from build123d import *

# Parameters (mm, degrees)
SKETCH3_R           = 145
SKETCH3_R_2         = 105
BOSS_EXTRUDE1_START = -50
SKETCH4_W           = 360
SKETCH4_H           = 360
SKETCH4_R           = 145
BOSS_EXTRUDE1_DEPTH = 50
FILLET1_R           = 20
SKETCH6_W           = 360
SKETCH6_H           = 360
SKETCH6_R           = 145
BOSS_EXTRUDE2_DEPTH = 50
FILLET2_R           = 20
SKETCH7_R           = 30
BOSS_EXTRUDE4_DEPTH = 10


with BuildPart() as part:
    # Sweep-Thin1: sweep along a path in Sketch2
    with BuildLine(Plane.XY) as sweep_thin1_path:
        Line((0, 0), (-150, 0))
        ThreePointArc((-150, 0), (-333.847763109, 76.152236891), (-410, 260))
        Line((-410, 260), (-410, 410))
    # Sketch3 → Sweep-Thin1 (sweep)
    with BuildSketch(Plane(origin=(0, 0, 0), x_dir=(0, 0, -1), z_dir=(1, 0, 0))):
        Circle(SKETCH3_R)
        Circle(SKETCH3_R_2, mode=Mode.SUBTRACT)
    sweep(path=sweep_thin1_path.line)

    # Sketch4 → Boss-Extrude1 (add)
    with BuildSketch(Plane(origin=(0, 0, 0), x_dir=(0, 0, -1), z_dir=(1, 0, 0)).offset(BOSS_EXTRUDE1_START)):
        Rectangle(SKETCH4_W, SKETCH4_H)
        with Locations(Location((0, 0, 0), (0, 0, 270))):
            Circle(SKETCH4_R, mode=Mode.SUBTRACT)
    extrude(amount=BOSS_EXTRUDE1_DEPTH)

    # Fillet1
    fillet1_edges = [part.edges().sort_by_distance(p)[0] for p in [
        (-25, -180, -180),
        (-25, -180, 180),
        (-25, 180, 180),
        (-25, 180, -180),
    ]]
    fillet(fillet1_edges, radius=FILLET1_R)

    # Sketch6 → Boss-Extrude2 (add)
    with BuildSketch(Plane(origin=(0, 410, 0), x_dir=(1, 0, 0), z_dir=(0, 1, 0))):
        with Locations((-410, 0)):
            Rectangle(SKETCH6_W, SKETCH6_H)
        with Locations(Location((-410, 0, 0), (0, 0, 180))):
            Circle(SKETCH6_R, mode=Mode.SUBTRACT)
    extrude(amount=-BOSS_EXTRUDE2_DEPTH)

    # Fillet2
    fillet2_edges = [part.edges().sort_by_distance(p)[0] for p in [
        (-230, 385, 180),
        (-590, 385, 180),
        (-590, 385, -180),
        (-230, 385, -180),
    ]]
    fillet(fillet2_edges, radius=FILLET2_R)

    # Sketch7 → Boss-Extrude4 (add)
    with BuildSketch(Plane(origin=(0, 0, 0), x_dir=(0, 0, -1), z_dir=(1, 0, 0))):
        with Locations((-130, 130)):
            Circle(SKETCH7_R)
    extrude(amount=-BOSS_EXTRUDE4_DEPTH)


solid = part.part
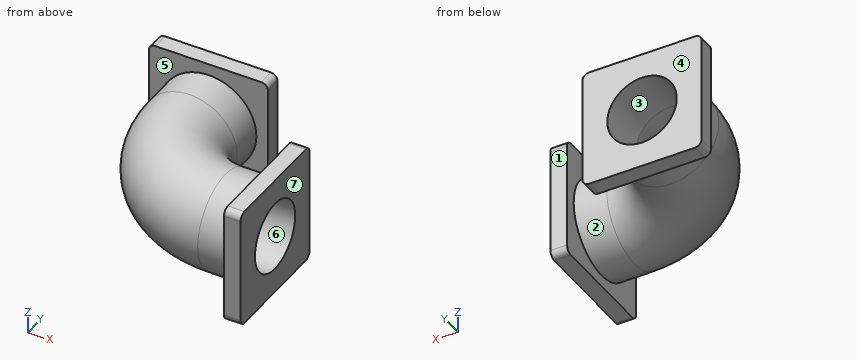
Can you work these out from the model? Positions are in its coordinate system, mm. Face numbers are marked on the shaded views. A direction names the side the tool comes from. Round coordinates to 2 decimals unless told otherwise and drop trailing zeros. Order: outer loops, then holes, each group sorted by start corner. A loop starts at its lowest first (then second) coordinate and runs counter-clockwise, first axis right, second up. Notation, with made-up numbers: (87.5, -33) -> (96.5, -33) arc R14 cw to (96.5, -17) -> close; hole circle Ø3 at (46.5, -38). An arc over 180 degrees is marked (long way). Write each question's results on one line, items separated by ' | '. Start each with the question number.
Item 1: Which directions (+Z, -Z, +X, -X, +Y, -Y) give clear straight access to the entire face, cutting with the end or side of a thin tool? Please do the marked faces 1, 2 and 3.
Item 2: Will these pins go through, and if not, where does the flat tip stop? pin 1 (12 mm diameter, centred on y = 26, z = 20, fed in from -X); pin 2 (1.5 mm diameter, centred on x = -424, y = 247, fed in from -Z); pin 3 (10 mm diameter, centred on x = -359, y = 231, fed in from -Z).
Item 3: Please list where these lines run through material, in increasing order: L1, parallel to Y at x = -93, z = 0; L2, parallel to X at y = 325.5, z = 0.
Item 4: Thinking about a two-plate mould opening in Y: for the marked faces 4, 5, 6 and 7, which applies, +Y half, -Y half, draft (parallel to the pull), parting line (faces both ways), or undercut?
Item 5: If we section it at A-A, the plane z = 0: Write out the boundary of the cut face in (x, y).
Results:
1) face 1: +Z, -Z, +X, +Y | face 2: none | face 3: +Y
2) pin 1: stops at x = -483.16 | pin 2: stops at z = -144.36 | pin 3: stops at z = -138.16
3) L1: y = -145 to -105, 105 to 145 | L2: x = -555 to -515, -305 to -265
4) face 4: +Y half | face 5: undercut | face 6: undercut | face 7: draft
5) outline: (-590, 360) -> (-555, 360) -> (-555, 260) arc R405 ccw to (-150, -145) -> (-50, -145) -> (-50, -180) -> (0, -180) -> (0, -105) -> (-150, -105) arc R365 cw to (-515, 260) -> (-515, 410) -> (-590, 410) -> close; (-305, 260) arc R155 ccw to (-150, 105) -> (0, 105) -> (0, 180) -> (-50, 180) -> (-50, 145) -> (-150, 145) arc R115 cw to (-265, 260) -> (-265, 360) -> (-230, 360) -> (-230, 410) -> (-305, 410) -> close
